The listing builds one solid part. Answer for the finished solid, in the listing's coordinates (mm). Face numbers are marked on the shaded views. A direction names the side the tool comes from. Give positions to 0.01 mm unless a question says otherwise; leave off trailing zeros. Order: outer loops, then holes, each group sorted by start corner. A loop starts at its lowest first (then second) coordinate and runs counter-clockwise, first axis right, second up. Notation, with made-up numbers: (16.25, 87.25) - (23.25, 87.25) arc R26 cw to (23.25, 123.25) - close; hole circle Ø3 at (-31.75, 79). An arc over 180 degrees is marked (long way). Answer as CSV lines item,"result". Start each with the question number.
1. Consider line 1 along Z through (x, y) = (12, 1.65); line 2 along X through (y, z) = (2.5, 6.25); line 3 along X through (y, z) = (1.25, 0.25). Determine where each line is inside the solid, lowest interval first. Write a range as [from, to].
2. Section A-A on z = 0 is taken. Give the vertices of the cut face in (x, y), and give its area (3 significant figures).
3. Flat-ended cylindrical pins translate along their axes: pin 1 (2.5 mm diameter, centred on x = -5.5, z = 0, fed in from -Y); pin 2 (1.5 mm diameter, centred on x = -0.5, y = 0.5, fed in from +Z); pin 3 (0.9 mm diameter, centred on y = 1, z = -8.5, fed in from +X). Find the tip coordinate at first contact, or state that the pin passes through.
4. Which of the six approach directions +Z, -Z, +X, -X, +Y, -Y give full straight-line access (tool end or side, diameter ignored) to the marked faces 4, 5 and 6?
5. Section C-C on x = 12 is taken. Give the vertices of the cut face in (y, z), and give its area (3 significant figures).
6. Section B-B on y = 1 is taken. Give the vertices of the cut face in (x, z).
7. Determine the mould class of the marked faces 1, 2 and 3 for opening direction X: +X half, -X half, draft (parallel to the pull), parting line (faces both ways), or undercut.
8. Section D-D on x = -10.5 is taken. Give the vertices of the cut face in (y, z), and give its area (3 significant figures).
Autodesk Inventor part; units mm, degrees
ref_plane "YZ Plane" through (0, 0, 0) normal (1, 0, 0) x (0, 1, 0)
ref_plane "XZ Plane" through (0, 0, 0) normal (0, 1, 0) x (-1, 0, 0)
ref_plane "XY Plane" through (0, 0, 0) normal (0, 0, 1) x (1, 0, 0)
sketch "Sketch1" plane through (0, 0, 0) normal (0, 1, 0) x (-1, 0, 0)
  line L0 (16, 10) -> (-16, 10)
  line L1 (-16, 10) -> (-16, -10)
  line L2 (-16, -10) -> (16, -10)
  line L3 (16, -10) -> (16, 10)
  line L4 (16, 10) -> (-16, -10) construction
  line L5 (-16, 10) -> (16, -10) construction
  line L6 (-16, -10) -> (11, -10)
  line L7 (11, -10) -> (11, -5)
  line L8 (11, -5) -> (-16, -5)
  line L9 (-16, -5) -> (-16, -10)
  line L10 (-16, 10) -> (11, 10)
  line L11 (11, 10) -> (11, 5)
  line L12 (11, 5) -> (-16, 5)
  line L13 (-16, 5) -> (-16, 10)
  line L14 (11, 0) -> (8, 0)
  line L15 (8, 0) -> (5.5, 0)
  line L16 (5.5, 0) -> (-12, 0)
  circle A0 centre (5.5, 0) radius 1.5
  circle A1 centre (-12, 0) radius 1.5
  point P0 (0, 0)
  dimension "d0" = 32
  dimension "d1" = 20
  dimension "d2" = 27
  dimension "d3" = 5
  dimension "d4" = 27
  dimension "d5" = 5
  dimension "d6" = 3
  dimension "d7" = 2.5
  dimension "d8" = 17.5
  dimension "d9" = 3
  dimension "d10" = 3
  dimension "d13" = 10
extrude "Extrusion1" add sketch "Sketch1" along normal blind 3 contours L3 L2 L7 L8 L1 L12 L11 L0
sketch "Sketch2" plane through (0, 3, 0) normal (0, 1, 0) x (1, 0, 0)
  point P0 (0, 0)
properties part number "Stand T Sd Serayu 2024"
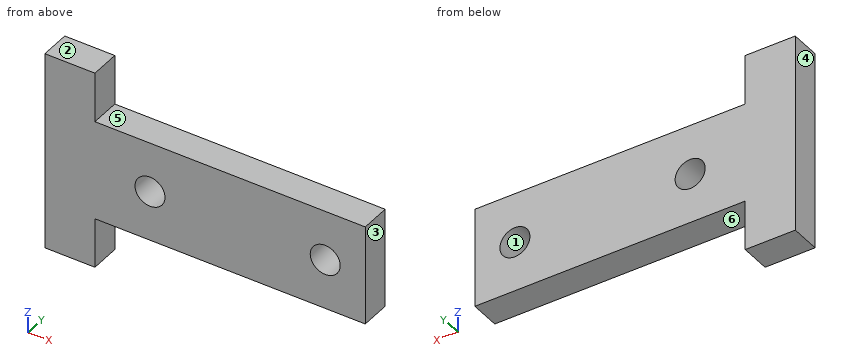
Checks:
1,line 1,"z = [-5, -1.5], [1.5, 5]"
1,line 2,"x = [-16, -11]"
1,line 3,"x = [-16, -6.98], [-4.02, 10.52], [13.48, 16]"
2,outline,"(-16, 0) - (-7, 0) - (-7, 3) - (-16, 3) - close; (-4, 0) - (10.5, 0) - (10.5, 3) - (-4, 3) - close; (13.5, 0) - (16, 0) - (16, 3) - (13.5, 3) - close"
2,area,"78.0 mm²"
3,pin 1,"passes through"
3,pin 2,"stops at z = 5"
3,pin 3,"stops at x = -11"
4,face 4,"+Z, -Z, -X, +Y, -Y"
4,face 5,"+Z, +X, +Y, -Y"
4,face 6,"-Z, +X, +Y, -Y"
5,outline,"(0, -5) - (3, -5) - (3, -1.5) - (0, -1.5) - close; (0, 1.5) - (3, 1.5) - (3, 5) - (0, 5) - close"
5,area,"21.0 mm²"
6,outline,"(-16, -10) - (-11, -10) - (-11, -5) - (16, -5) - (16, 5) - (-11, 5) - (-11, 10) - (-16, 10) - close; hole circle Ø3 at (-5.5, 0); hole circle Ø3 at (12, 0)"
7,face 1,"undercut"
7,face 2,"draft"
7,face 3,"+X half"
8,outline,"(0, -5) - (3, -5) - (3, 5) - (0, 5) - close"
8,area,"30.0 mm²"
